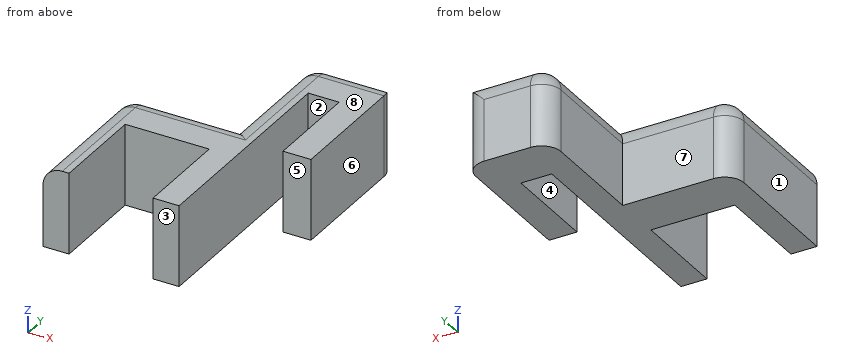
Autodesk Inventor part; units mm, degrees
ref_plane "YZ Plane" through (0, 0, 0) normal (1, 0, 0) x (0, 1, 0)
ref_plane "XZ Plane" through (0, 0, 0) normal (0, 1, 0) x (-1, 0, 0)
ref_plane "XY Plane" through (0, 0, 0) normal (0, 0, 1) x (1, 0, 0)
sketch "Sketch1" plane through (0, 0, 0) normal (0, 0, 1) x (1, 0, 0)
  line L0 (0, 0) -> (-8.7, 0)
  line L1 (-8.7, 0) -> (-8.7, 8.7)
  line L2 (-8.7, 8.7) -> (0, 8.7)
  line L3 (0, 8.7) -> (0, 0)
  dimension "d0" = 8.7
  dimension "d1" = 8.7
extrude "Extrusion1" [suppressed]
sketch "Sketch2" plane through (-8.7, 0, 0) normal (-1, 0, 0) x (0, 0, 1)
  line L0 (0, 8.7) -> (0, 0)
  line L1 (0, 0) -> (3, 0)
  line L2 (3, 0) -> (3, 8.7)
  line L3 (3, 8.7) -> (0, 8.7)
  line L4 (0, 8.7) -> (0, 0)
extrude "Extrusion2" [suppressed]
sketch "Sketch3" plane through (0, 0, 3) normal (0, 0, 1) x (1, 0, 0)
  line L0 (0, 8.7) -> (-11.7, 8.7)
  line L1 (0, 0) -> (-11.7, 0)
  line L2 (-11.7, 8.7) -> (-8.7, 8.7)
  line L3 (-8.7, 8.7) -> (-8.7, 0)
  line L4 (-8.7, 0) -> (-11.7, 0)
  line L5 (-11.7, 0) -> (-11.7, 8.7)
  dimension "d6" = 3
extrude "Extrusion3" [suppressed]
sketch "Sketch5" plane through (0, 0, 0) normal (1, 0, 0) x (0, 0, -1)
  line L0 (0, 8.7) -> (-3, 8.7)
  line L1 (0, 0) -> (-3, 0)
  line L2 (-3, 0) -> (-3, 8.7)
  line L3 (-3, 8.7) -> (0, 8.7)
  line L4 (0, 8.7) -> (0, 0)
  dimension "d9" = 3
extrude "Extrusion4" [suppressed]
sketch "Sketch6" plane through (0, 0, 3) normal (0, 0, 1) x (1, 0, 0)
  line L0 (3, 8.7) -> (-11.7, 8.7)
  line L1 (3, 8.7) -> (0, 8.7)
  line L2 (0, 8.7) -> (0, 0)
  line L3 (0, 0) -> (3, 0)
  line L4 (3, 0) -> (3, 8.7)
extrude "Extrusion5" [suppressed]
sketch "Sketch7" plane through (0, 0, 0) normal (0, 0, 1) x (1, 0, 0)
  line L0 (0, 0) -> (-2.7, 0)
  line L1 (-2.7, 0) -> (-2.7, 15)
  line L2 (-2.7, 15) -> (0, 15)
  line L3 (0, 15) -> (0, 0)
  line L4 (-2.7, 15) -> (-11.4, 15)
  line L5 (-11.4, 15) -> (-11.4, 10)
  line L6 (-11.4, 10) -> (-2.7, 10)
  line L7 (-2.7, 10) -> (-2.7, 15)
  line L8 (-11.4, 15) -> (-14.1, 15)
  line L9 (-14.1, 15) -> (-14.1, 0)
  line L10 (-14.1, 0) -> (-11.4, 0)
  line L11 (-11.4, 0) -> (-11.4, 15)
  line L12 (-2.7, 15) -> (0, 15)
  line L13 (0, 15) -> (0, 23)
  line L14 (0, 23) -> (-2.7, 23)
  line L15 (-2.7, 23) -> (-2.7, 15)
  line L16 (-2.7, 23) -> (0, 23)
  line L17 (0, 23) -> (0, 28)
  line L18 (0, 28) -> (-2.7, 28)
  line L19 (-2.7, 28) -> (-2.7, 23)
  line L20 (0, 28) -> (3.2, 28)
  line L21 (3.2, 28) -> (3.2, 23)
  line L22 (3.2, 23) -> (0, 23)
  line L23 (0, 23) -> (0, 28)
  line L24 (3.2, 28) -> (6.1, 28)
  line L25 (6.1, 28) -> (6.1, 23)
  line L26 (6.1, 23) -> (3.2, 23)
  line L27 (3.2, 23) -> (3.2, 28)
  line L28 (6.1, 23) -> (3.2, 23)
  line L29 (3.2, 23) -> (3.2, 13)
  line L30 (3.2, 13) -> (6.1, 13)
  line L31 (6.1, 13) -> (6.1, 23)
  point P0 (-11.4, 10)
  point P1 (-2.7, 10)
  dimension "d14" = 2.7
  dimension "d15" = 15
  dimension "d16" = 8.7
  dimension "d17" = 5
  dimension "d18" = 2.7
  dimension "d19" = 15
  dimension "d23" = 2.7
  dimension "d24" = 8
  dimension "d25" = 5
  dimension "d26" = 3.2
  dimension "d27" = 5
  dimension "d28" = 2.9
  dimension "d29" = 2.9
  dimension "d30" = 10
extrude "Extrusion6" add sketch "Sketch7" along normal blind 8.4
fillet "Fillet1" radius 2 3 edges at (-14.1, 7.5, 8.4) (-8.4, 15, 8.4) (-14.1, 15, 4.2)
fillet "Fillet2" radius 2 4 edges at (-2.7, 21.5, 8.4) (1.7, 28, 8.4) (6.1, 28, 4.2) (-2.7, 28, 4.2)
properties part number "Hook_TestFit"
Here's how the part is built. I have some questions about the finished solid (model axes, mm). Face numbers are marked on the shaded views. A direction names the side the tool comes from. Give positions to 0.01 mm unless a question says otherwise; leave off trailing zeros. Order: outer loops, then holes, each group sorted by start corner. A loop starts at its lowest first (then second) coordinate and runs counter-clockwise, first axis right, second up. Notation, with made-up numbers: (40.5, 74.5) -> (58.5, 74.5) arc R24 cw to (58.5, 91.5) -> close; hole circle Ø8 at (81, 29.5). An arc over 180 degrees is marked (long way). Use a Markdown table: item, result. Add a question column.
Item 1: For the marked faces 4, 5, 6, 7 and 8, which set-ups out of +Z, -Z, +X, -X, +Y, -Y let a thin tool reach every point of the face, with its end or its side?
Item 2: Imagine slicing it at A-A on y = 2.25. Please give me the cut outline in (x, z), plus the area to 3 significant figures.
Item 3: Will these pins go through, and if not, where does the flat tip stop? pin 1 (4 mm diameter, centred on x = -8.5, z = 5, fed in from -Y); pin 2 (1 mm diameter, centred on x = 2.5, z = 3, fed in from -Y); pin 3 (1.9 mm diameter, centred on y = 19, z = 2, fed in from -X).
Item 4: If we mould it in two halves opening along X, with no side actions, what happens to the marked faces 1, 2 and 3? For each: pulls with the +X half, pulls with the -X half, needs draft (parallel to the pull), parting line crosses it, or undercut.
Item 5: Imagine slicing it at B-B on y = 20.25. Please give me the cut outline in (x, z), plus the area to 3 significant figures.
Item 6: Imagine slicing it at D-D on x = -11. Please give me the cut outline in (y, z), plus the area to 3 significant figures.
Item 7: I need wall thicknesses on line 1 (X direction, y = 4.5, z = 3); line 2 (X direction, y = 19.25, z = 6.25); line 3 (Y direction, x = 1, z = 6.5). Which ranges of each line are inside material? Lowest first, please.
Item 8: Imagine slicing it at C-C on z = 0.5. Please give me the cut outline in (x, y).
Data:
| question | item | result |
|---|---|---|
| 1 | face 4 | +Z, -Z, -Y |
| 1 | face 5 | +Z, -Z, +X, -Y |
| 1 | face 6 | +Z, -Z, +X, +Y, -Y |
| 1 | face 7 | +Z, -Z, -X, +Y |
| 1 | face 8 | +Z, +X, -X, +Y, -Y |
| 2 | outline | (-14.1, 0) -> (-11.4, 0) -> (-11.4, 8.4) -> (-12.1, 8.4) arc R2 ccw to (-14.1, 6.4) -> close; (-2.7, 0) -> (0, 0) -> (0, 8.4) -> (-2.7, 8.4) -> close |
| 2 | area | 44.5 mm² |
| 3 | pin 1 | stops at y = 10 |
| 3 | pin 2 | stops at y = 23 |
| 3 | pin 3 | stops at x = -2.7 |
| 4 | face 1 | pulls with the -X half |
| 4 | face 2 | undercut |
| 4 | face 3 | needs draft |
| 5 | outline | (-2.7, 0) -> (0, 0) -> (0, 8.4) -> (-0.7, 8.4) arc R2 ccw to (-2.7, 6.4) -> close; (3.2, 0) -> (6.1, 0) -> (6.1, 8.4) -> (3.2, 8.4) -> close |
| 5 | area | 46.2 mm² |
| 6 | outline | (10, 0) -> (15, 0) -> (15, 6.4) arc R2 ccw to (13, 8.4) -> (10, 8.4) -> close |
| 6 | area | 41.1 mm² |
| 7 | line 1 | x = -14.1 to -11.4, -2.7 to 0 |
| 7 | line 2 | x = -2.7 to 0, 3.2 to 6.1 |
| 7 | line 3 | y = 23 to 28 |
| 8 | outline | (-14.1, 0) -> (-11.4, 0) -> (-11.4, 10) -> (-2.7, 10) -> (-2.7, 0) -> (0, 0) -> (0, 23) -> (3.2, 23) -> (3.2, 13) -> (6.1, 13) -> (6.1, 26) arc R2 ccw to (4.1, 28) -> (-0.7, 28) arc R2 ccw to (-2.7, 26) -> (-2.7, 15) -> (-12.1, 15) arc R2 ccw to (-14.1, 13) -> close |
